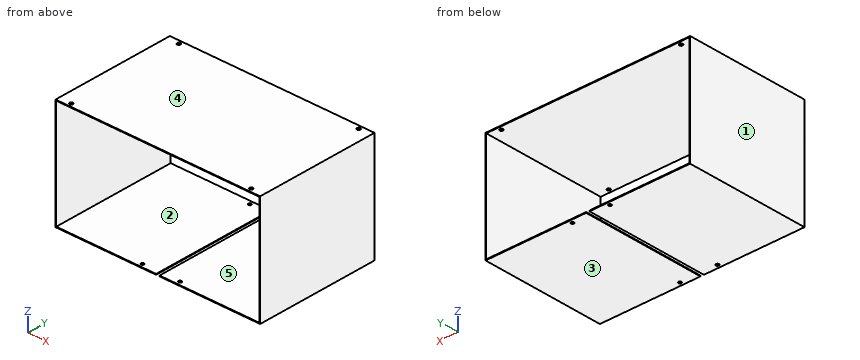
from build123d import *

# Parameters (mm, degrees)
F1_DEPTH = 165
F2_R     = 2
F3_DEPTH = 1
F4_R     = 2.25
F5_DEPTH = 1


with BuildPart() as f1:
    # F0 (on Front) → F1 (new body)
    with BuildSketch(Plane.XZ):
        Polygon((136.25, 72.75), (-136.25, 72.75), (-136.25, -72.75), (-2.25, -72.75), (-2.25, -71.75), (-135.25, -71.75), (-135.25, 71.75), (135.25, 71.75), (135.25, -71.75), (2.25, -71.75), (2.25, -72.75), (136.25, -72.75), align=None)
    extrude(amount=F1_DEPTH)

    # F2 (on face) → F3 (cut, through all)
    with BuildSketch(Plane(origin=(0, 0, -72.75), x_dir=(1, 0, 0), z_dir=(0, 0, -1))):
        with Locations((25, 160)):
            Circle(F2_R)
        with Locations((-25, 160)):
            Circle(F2_R)
        with Locations((25, 5)):
            Circle(F2_R)
        with Locations((-25, 5)):
            Circle(F2_R)
    extrude(amount=-F3_DEPTH, mode=Mode.SUBTRACT)

    # F4 (on face) → F5 (cut, through all)
    with BuildSketch(Plane.XY.offset(72.75)):
        with Locations((-119.75, -5)):
            Circle(F4_R)
        with Locations((119.75, -5)):
            Circle(F4_R)
        with Locations((-119.75, -160)):
            Circle(F4_R)
        with Locations((119.75, -160)):
            Circle(F4_R)
    extrude(amount=-F5_DEPTH, mode=Mode.SUBTRACT)


solid = f1.part
CAD build for the part. Positions are in the model's coordinates, mm. Face numbers are marked on the shaded views. A direction names the side the tool comes from. Coordinates: 2 decimals unless noted, no trailing zeros. Loops run counter-clockwise (first coordinate to the right, second up) from the corner with the lowest first, then second, coordinate; pieces in that order, holes last. Notation, with made-up numbers: (60.5, 16.5) -> (115.5, 16.5) arc R16 cw to (115.5, 46.5) -> close; hole circle Ø10 at (-40, -26.75). An arc over 180 degrees is marked (long way). One line per item, written item: value.
1. Flat gauge pin, fed straight in: P1, Ø3.5, axis at x = -25, y = -160, coming from the -Z side. Where does the tip first touch, or does it go through?
Answers:
P1: stops at z = 71.75
2. Slice it at A-A on x = 106. Write the cut outline in (y, z).
Answers:
outline: (-165, -72.75) -> (0, -72.75) -> (0, -71.75) -> (-165, -71.75) -> close; (-165, 71.75) -> (0, 71.75) -> (0, 72.75) -> (-165, 72.75) -> close
3. Pull direction Z, two halves, no side cores. Call the marked faces 3, 4 and 5: pulls with the +Z half, pulls with the -Z half, needs draft (parallel to the pull), parting line crosses it, or undercut.
Answers:
face 3: pulls with the -Z half
face 4: pulls with the +Z half
face 5: undercut
4. Drill centre lines: line 1 (Y direction, x = 25, z = -72.3); line 2 (X direction, y = -160, z = 72.3); line 3 (X direction, y = -160, z = -72.3). Where is each one in solid material? Low to high. Write a range as [from, to].
Answers:
line 1: y = [-165, -162], [-158, -7], [-3, 0]
line 2: x = [-136.25, -122], [-117.5, 117.5], [122, 136.25]
line 3: x = [-136.25, -27], [-23, -2.25], [2.25, 23], [27, 136.25]
5. Slice it at B-B on z = 34. Write the cut outline in (x, y).
Answers:
outline: (-136.25, -165) -> (-135.25, -165) -> (-135.25, 0) -> (-136.25, 0) -> close; (135.25, -165) -> (136.25, -165) -> (136.25, 0) -> (135.25, 0) -> close
6. Which spindle directions (+Z, -Z, +X, -X, +Y, -Y) get a long thin tool onto all of the face, cutting with end or side? Do the marked faces 1 and 2. Say none if no direction does.
Answers:
face 1: +Z, -Z, -X, +Y, -Y
face 2: +Y, -Y
7. Slice it at C-C on y = -89. Write the cut outline in (x, z).
Answers:
outline: (-136.25, -72.75) -> (-2.25, -72.75) -> (-2.25, -71.75) -> (-135.25, -71.75) -> (-135.25, 71.75) -> (135.25, 71.75) -> (135.25, -71.75) -> (2.25, -71.75) -> (2.25, -72.75) -> (136.25, -72.75) -> (136.25, 72.75) -> (-136.25, 72.75) -> close
